Geometry: final body of the model. Coordinates: model frame, mm. A direction names the side the tool comes from. Coordinates: 2 decimals unless noted, no trailing zeros. Write each loop counter-clockwise with the first axis right and the second up, starting at its lowest first coordinate (ties: lowest second). Pieces come first, ordered by that corner, then holes. Notation, with made-up numbers: (5, -9) - (45, -9) arc R38 cw to (45, 30) - close; hole circle Ø11 at (19.5, 60). An arc over 180 degrees is marked (long way). Answer as a JSON object with one key per item and string values. Group by question number.
Item 1: Section C-C on x = 8. Return loops of the section in (y, z).
Item 2: Set-up query: faces 1 (the flat face through (8, 42, -1)), 2 (the flat face through (8, 20, 7)), 3 (the flat face through (15, 35.2, -0.7)). Return all of +Z, -Z, +X, -X, +Y, -Y with unobstructed straight access to the full face (end or side cutting, diameter ignored); none if empty.
Item 3: Section D-D on y = 5.5. Return loops of the section in (x, z), and give its area (3 significant figures).
Item 4: Section A-A on y = 41. Return loops of the section in (x, z).
Item 5: Line query: line 1 along Y through (x, z) = (3.25, 11.5); line 2 along Z through (x, y) = (12.5, 39.5); line 3 along X through (y, z) = (41.5, -2.5). Output: solid intervals per line, ascending. Write a range as from..to.
Item 6: First-contact query: pin 1 Ø7.5 at (y, z) = (39.5, -8) entering from +X; pin 2 Ø1.5 at (y, z) = (50.5, 1) entering from -X; pin 3 Ø0.6 at (y, z) = (19.5, 11) entering from -X; pin 4 Ø6 at (x, z) = (3.5, 4) entering from -Y. Flat tips, straight axial feed; report the tip coordinate or a pass-through.
Item 7: Section B-B on z = -9. Return loops of the section in (x, y).
```python
from build123d import *

# Parameters (mm, degrees)
EXTRUDE_1_DEPTH     = 65
CUT_EXTRUDE_START   = -20
SKETCH_6_W          = 14
SKETCH_6_H          = 1
CUT_EXTRUDE_2_DEPTH = 20
SKETCH_7_W          = 14
SKETCH_7_H          = 0.75
EXTRUDE_2_DEPTH     = 16


with BuildPart() as part:
    # Эскиз1 → Бобышка-Вытянуть1 (new body)
    with BuildSketch(Plane(origin=(0, 0, 0), x_dir=(1, 0, 0), z_dir=(0, 1, 0))):
        Polygon((0, 0), (0, 15), (1, 15), (1, 1), (15, 1), (15, 0), align=None)
    extrude(amount=EXTRUDE_1_DEPTH)

    # Эскиз6 → Вырез-Вытянуть2 (cut)
    with BuildSketch(Plane.XZ.offset(CUT_EXTRUDE_START)):
        with Locations((8, -0.5)):
            Rectangle(SKETCH_6_W, SKETCH_6_H)
    extrude(amount=CUT_EXTRUDE_2_DEPTH, mode=Mode.SUBTRACT)

    # Эскиз7 → Бобышка-Вытянуть2 (add)
    with BuildSketch(Plane(origin=(0, 0, -1), x_dir=(-1, 0, 0), z_dir=(0, 0, -1))):
        with Locations((-8, 19.625)):
            Rectangle(SKETCH_7_W, SKETCH_7_H)
    extrude(amount=-EXTRUDE_2_DEPTH)


solid = part.part
```
Checks:
{
 "1": {"outline": "(19.25, -1) - (65, -1) - (65, 0) - (20, 0) - (20, 15) - (19.25, 15) - close"},
 "2": {"face 1": "-Z, +X, +Y, -Y", "face 2": "+Z, +X, -X, +Y", "face 3": "+Z, -Z, +X, +Y, -Y"},
 "3": {"outline": "(0, -15) - (1, -15) - (1, 0) - (0, 0) - close", "area": "15.0 mm^2"},
 "4": {"outline": "(0, -15) - (1, -15) - (1, -1) - (15, -1) - (15, 0) - (0, 0) - close"},
 "5": {"line 1": "19.25..20", "line 2": "-1..0", "line 3": "0..1"},
 "6": {"pin 1": "x = 1", "pin 2": "through", "pin 3": "x = 1", "pin 4": "y = 19.25"},
 "7": {"outline": "(0, 0) - (1, 0) - (1, 65) - (0, 65) - close"}
}
